Design review of the part built by this model. Coordinates are the model's own, in mm. A direction names the side the tool comes from. Give positions to 0.01 mm unless a question says otherwise; leave off trailing zeros. Write each loop counter-clockwise with the first axis right and the second up, starting at its lowest first coordinate (ties: lowest second). Pieces come first, ordered by that corner, then holes.
```python
from build123d import *

# Parameters (mm, degrees)
SKETCH_W        = 18.4
SKETCH_H        = 10
PAD_DEPTH       = 8
SKETCH002_R     = 2.6
POCKET_DEPTH    = 10
SKETCH003_W     = 16
SKETCH003_H     = 8.8
POCKET001_DEPTH = 6.8
SKETCH004_W     = 10.8
SKETCH004_H     = 3
POCKET002_DEPTH = 5


with BuildPart() as part:
    # Sketch → Pad (new body)
    with BuildSketch(Plane.XY):
        Rectangle(SKETCH_W, SKETCH_H)
    extrude(amount=PAD_DEPTH)

    # Sketch002 (on Face3 of Pad) → Pocket (cut)
    with BuildSketch(Plane(origin=(0, 5, 0), x_dir=(-1, 0, 0), z_dir=(0, 1, 0))):
        with Locations((-5.4, 4)):
            Circle(SKETCH002_R)
        with Locations((0, 4)):
            Circle(SKETCH002_R)
        with Locations((5.4, 4)):
            Circle(SKETCH002_R)
    extrude(amount=-POCKET_DEPTH, mode=Mode.SUBTRACT)

    # Sketch003 (on Face4 of Pocket) → Pocket001 (cut)
    with BuildSketch(Plane.XY.offset(8)):
        with Locations((0, -0.6)):
            Rectangle(SKETCH003_W, SKETCH003_H)
    extrude(amount=-POCKET001_DEPTH, mode=Mode.SUBTRACT)

    # Sketch004 (on Face7 of Pocket001) → Pocket002 (cut)
    with BuildSketch(Plane(origin=(0, 5, 0), x_dir=(-1, 0, 0), z_dir=(0, 1, 0))):
        with Locations((0, 4)):
            Rectangle(SKETCH004_W, SKETCH004_H)
    extrude(amount=-POCKET002_DEPTH, mode=Mode.SUBTRACT)


solid = part.part
```
(1) Mouldability with a two-part tool opening along Z and no side actions: class faces 4 (the face through (0, -1, 1.2)), 5 (the face through (0, 4.4, 1.4)), 6 (the face through (-9.2, 0, 4)) as pulls with the +Z half, pulls with the -Z half, needs draft (parallel to the pull), parting line crosses it, or undercut.
Resolved:
face 4: pulls with the +Z half
face 5: undercut
face 6: needs draft
(2) Consider section B-B, the plane x = 5.4. Give the boundary of the cut face in (y, z), then the cut area to 3 significant figures.
Resolved:
outline: (-5, 0) - (5, 0) - (5, 1.4) - (3.8, 1.4) - (3.8, 1.2) - (-5, 1.2) - close; (3.8, 6.6) - (5, 6.6) - (5, 8) - (3.8, 8) - close
area: 13.9 mm2
(3) Clearance check with a flat-ended pin moving along its axis: P1, Ø3, axis at x = 2, z = 6, coming from the -Y side. State where the tip first meets the part, or that it passes through.
Resolved:
P1: stops at y = 3.8
(4) Tool access review of faces 1 (the face through (-3, 4, 2.5)), 2 (the face through (0, 5, 1)), 3 (the face through (-1.2, 3.8, 1.5)): name each direction out of +Z, -Z, +X, -X, +Y, -Y from which nothing blocks a thin tool from reaching the whole face with its end or side.
Resolved:
face 1: +Y, -Y
face 2: +Z, -Z, +X, -X, +Y
face 3: +Z, -Y
(5) Consider section C-C, the plane z = 4.5. Give the boundary of the cut face in (x, y).
Resolved:
outline: (-9.2, -5) - (-8, -5) - (-8, 3.8) - (-7.95, 3.8) - (-7.95, 5) - (-9.2, 5) - close; (7.95, 3.8) - (8, 3.8) - (8, -5) - (9.2, -5) - (9.2, 5) - (7.95, 5) - close
(6) Consider section D-D, the plane y = 1.5. Give the boundary of the cut face in (x, z).
Resolved:
outline: (-9.2, 0) - (9.2, 0) - (9.2, 8) - (8, 8) - (8, 1.2) - (-8, 1.2) - (-8, 8) - (-9.2, 8) - close
(7) To check wall thickness, follow L1, parallel to X at y = -0.5, z = 2.25; L2, parallel to Z at x = -5.4, y = 4.6; L3, parallel to Z at x = -1.75, y = -1.75. State the ranges of each line that lie inside material, in increasing order.
Resolved:
L1: x = -9.2 to -8, 8 to 9.2
L2: z = 0 to 1.4, 6.6 to 8
L3: z = 0 to 1.2
(8) Consider section A-A, the plane z = 2.25. Give the boundary of the cut face in (x, y).
Resolved:
outline: (-9.2, -5) - (-8, -5) - (-8, 3.8) - (-7.32, 3.8) - (-7.32, 5) - (-9.2, 5) - close; (-3.48, 3.8) - (-1.92, 3.8) - (-1.92, 5) - (-3.48, 5) - close; (1.92, 3.8) - (3.48, 3.8) - (3.48, 5) - (1.92, 5) - close; (7.32, 3.8) - (8, 3.8) - (8, -5) - (9.2, -5) - (9.2, 5) - (7.32, 5) - close
